The listing builds one solid part. Answer for the finished solid, in the listing's coordinates (mm). Coordinates: 2 decimals unless noted, no trailing zeros. Write each loop counter-clockwise with the first axis right and the second up, starting at its lowest first coordinate (ties: lowest second). Pieces come first, ordered by that corner, then holes.
```python
from build123d import *

# Parameters (mm, degrees)
F0_W     = 30
F0_H     = 30
F1_DEPTH = 1760
F2_R     = 7.5
F3_DEPTH = 30.001
F4_R     = 5


with BuildPart() as f1:
    # F0 (on Top) → F1 (new body)
    with BuildSketch(Plane.XY):
        Rectangle(F0_W, F0_H)
    extrude(amount=F1_DEPTH)

    # F2 (on face) → F3 (cut, through all)
    with BuildSketch(Plane.YZ.offset(15)):
        with Locations((0, 30)):
            Circle(F2_R)
        with Locations((0, 92)):
            Circle(F2_R)
        with Locations((0, 154)):
            Circle(F2_R)
        with Locations((0, 216)):
            Circle(F2_R)
        with Locations((0, 278)):
            Circle(F2_R)
        with Locations((0, 340)):
            Circle(F2_R)
        with Locations((0, 402)):
            Circle(F2_R)
        with Locations((0, 464)):
            Circle(F2_R)
        with Locations((0, 526)):
            Circle(F2_R)
        with Locations((0, 588)):
            Circle(F2_R)
        with Locations((0, 650)):
            Circle(F2_R)
        with Locations((0, 712)):
            Circle(F2_R)
        with Locations((0, 774)):
            Circle(F2_R)
        with Locations((0, 836)):
            Circle(F2_R)
        with Locations((0, 898)):
            Circle(F2_R)
        with Locations((0, 960)):
            Circle(F2_R)
        with Locations((0, 1022)):
            Circle(F2_R)
        with Locations((0, 1084)):
            Circle(F2_R)
        with Locations((0, 1146)):
            Circle(F2_R)
        with Locations((0, 1208)):
            Circle(F2_R)
        with Locations((0, 1270)):
            Circle(F2_R)
        with Locations((0, 1332)):
            Circle(F2_R)
        with Locations((0, 1394)):
            Circle(F2_R)
        with Locations((0, 1456)):
            Circle(F2_R)
        with Locations((0, 1518)):
            Circle(F2_R)
        with Locations((0, 1580)):
            Circle(F2_R)
        with Locations((0, 1642)):
            Circle(F2_R)
        with Locations((0, 1704)):
            Circle(F2_R)
    extrude(amount=-F3_DEPTH, mode=Mode.SUBTRACT)

    # F4
    f4_edges = [f1.edges().sort_by_distance(p)[0] for p in [
        (15, -15, 880),
        (-15, -15, 880),
        (15, 15, 880),
        (-15, 15, 880),
    ]]
    fillet(f4_edges, radius=F4_R)


solid = f1.part
```
(1) Section A-A, the plane x = -5 is taken. State how many separate pieces and enclosed holes the cut face has, plus the area to 3 significant figures.
(2) Section B-B, the plane z = 1310 is taken. Write down the section's boundary in (x, y), plus the area to 3 significant figures.
(3) Find the intervals of material crossed by probe 1 along Y at (x, z) = (-8, 712); probe 2 along Y at (x, z) = (-2, 589.5); probe 3 along X at (y, z) = (-11.5, 769), in increasing order.
Solution:
1. separate pieces: 1
1. enclosed holes: 28
1. area: 47,900 mm2
2. outline: (-15, -10) arc R5 ccw to (-10, -15) - (10, -15) arc R5 ccw to (15, -10) - (15, 10) arc R5 ccw to (10, 15) - (-10, 15) arc R5 ccw to (-15, 10) - close
2. area: 879 mm2
3. probe 1: y = -15 to -7.5, 7.5 to 15
3. probe 2: y = -15 to -7.35, 7.35 to 15
3. probe 3: x = -14.77 to 14.77
